Model file for the job. Use its own axes, mm. Face numbers are marked on the shaded views. A direction names the side the tool comes from. Give positions to 0.01 mm unless a question says otherwise; leave off trailing zeros. Loops run counter-clockwise (first coordinate to the right, second up) from the corner with the lowest first, then second, coordinate; pieces in that order, holes last. Notation, with made-up numbers: (-26.5, 46) - (17.5, 46) arc R16 cw to (17.5, 62) - close; hole circle Ø5 at (1, 59). An arc over 180 degrees is marked (long way). Answer as CSV lines item,"result". Start each with the question number.
Item 1: Pin check, flat tips, straight feed: pin 1 (3 mm diameter, centred on y = -2, z = -4.5, fed in from -X); pin 2 (4 mm diameter, centred on x = 16.5, y = -0.5, fed in from +Z); pin 3 (1 mm diameter, centred on y = -2, z = 3, fed in from +X). Stop position of each tip, or through.
Item 2: Drill centre lines: L1, parallel to X at y = -3.5, z = 3.75; L2, parallel to Y at x = 17.75, z = 1.25; L3, parallel to X at y = -12.5, z = -5.25. Where is each one in solid material? Low to high. Write a range as from..to.
Item 3: Tool access for the marked faces 4, 5, 6 and 7: list every direction of +Z, -Z, +X, -X, +Y, -Y with a clear straight run to the whole face (end or side of a thin tool).
Item 4: Pull direction Z, two halves, no side cores. Call the marked faces 1, 2 and 3: pulls with the +Z half, pulls with the -Z half, needs draft (parallel to the pull), parting line crosses it, or undercut.
Item 5: Saw through at A-A on y = -11.5. Give the cut face in (x, z), plus the area to 3 significant figures.
Item 6: Saw through at C-C on z = 3. Give the cut face in (x, y), plus the area to 3 significant figures.
Item 7: Saw through at B-B on x = 17.75. Give the cut face in (y, z).
Item 8: Saw through at D-D on y = 0. State how many separate pieces and enclosed holes the cut face has, plus the area to 3 significant figures.
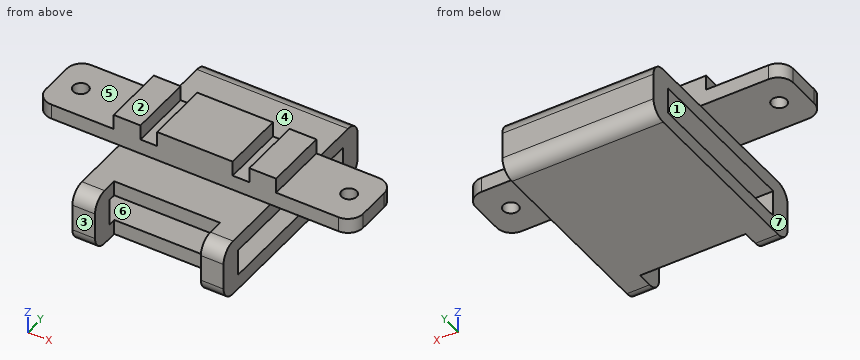
from build123d import *

# Parameters (mm, degrees)
SKETCH2_W           = 42
SKETCH2_H           = 8.4
BOSS_EXTRUDE1_DEPTH = 2
SKETCH3_W           = 3.55
SKETCH3_H           = 8.4
SKETCH3_W_2         = 10
BOSS_EXTRUDE2_DEPTH = 2
FILLET1_R           = 2
SKETCH4_R           = 1
CUT_EXTRUDE1_DEPTH  = 2
SKETCH5_W           = 20
SKETCH5_H           = 28
BOSS_EXTRUDE3_DEPTH = 7.5
FILLET2_R           = 2
SKETCH6_W           = 3.5
SKETCH6_H           = 22
CUT_EXTRUDE2_DEPTH  = 20
SKETCH7_W           = 14
SKETCH7_H           = 4
CUT_EXTRUDE3_DEPTH  = 10


with BuildPart() as part:
    # Sketch2 → Boss-Extrude1 (new body)
    with BuildSketch(Plane.XY):
        Rectangle(SKETCH2_W, SKETCH2_H)
    extrude(amount=BOSS_EXTRUDE1_DEPTH)

    # Sketch3 → Boss-Extrude2 (add)
    with BuildSketch(Plane.XY.offset(2)):
        with Locations((-8.975, 0)):
            Rectangle(SKETCH3_W, SKETCH3_H)
        with Locations((8.975, 0)):
            Rectangle(SKETCH3_W, SKETCH3_H)
        Rectangle(SKETCH3_W_2, SKETCH3_H)
    extrude(amount=BOSS_EXTRUDE2_DEPTH)

    # Fillet1
    fillet1_edges = [part.edges().sort_by_distance(p)[0] for p in [
        (-21, 4.2, 1),
        (21, 4.2, 1),
        (21, -4.2, 1),
        (-21, -4.2, 1),
    ]]
    fillet(fillet1_edges, radius=FILLET1_R)

    # Sketch4 → Cut-Extrude1 (cut)
    with BuildSketch(Plane.XY.offset(2)):
        with Locations((-17.75, 0)):
            Circle(SKETCH4_R)
        with Locations((17.75, 0)):
            Circle(SKETCH4_R)
    extrude(amount=-CUT_EXTRUDE1_DEPTH, mode=Mode.SUBTRACT)

    # Sketch5 → Boss-Extrude3 (add)
    with BuildSketch(Plane(origin=(0, 0, 0), x_dir=(-1, 0, 0), z_dir=(0, 0, -1))):
        Rectangle(SKETCH5_W, SKETCH5_H)
    extrude(amount=BOSS_EXTRUDE3_DEPTH)

    # Fillet2
    fillet2_edges = [part.edges().sort_by_distance(p)[0] for p in [
        (0, 14, 0),
        (0, -14, 0),
        (0, 14, -7.5),
        (0, -14, -7.5),
    ]]
    fillet(fillet2_edges, radius=FILLET2_R)

    # Sketch6 → Cut-Extrude2 (cut)
    with BuildSketch(Plane.ZY.offset(10)):
        with Locations((-3.75, 0)):
            Rectangle(SKETCH6_W, SKETCH6_H)
    extrude(amount=-CUT_EXTRUDE2_DEPTH, mode=Mode.SUBTRACT)

    # Sketch7 → Cut-Extrude3 (cut)
    with BuildSketch(Plane.XY):
        with Locations((0, -12)):
            Rectangle(SKETCH7_W, SKETCH7_H)
    extrude(amount=-CUT_EXTRUDE3_DEPTH, mode=Mode.SUBTRACT)


solid = part.part
Responses:
1,pin 1,"x = -10"
1,pin 2,"z = 2"
1,pin 3,"x = 10.75"
2,L1,"-10.75..-7.2, -5..5, 7.2..10.75"
2,L2,"-4.2..-1, 1..4.2"
2,L3,"-10..-7, 7..10"
3,face 4,"+Z, +X, -X, +Y"
3,face 5,"+Z, -X, +Y, -Y"
3,face 6,"+X, -X"
3,face 7,"-Z, -X, +Y, -Y"
4,face 1,"undercut"
4,face 2,"pulls with the +Z half"
4,face 3,"needs draft"
5,outline,"(-10, -7.5) - (-7, -7.5) - (-7, 0) - (-10, 0) - close; (7, -7.5) - (10, -7.5) - (10, 0) - (7, 0) - close"
5,area,"45.0 mm2"
6,outline,"(-10.75, -4.2) - (-7.2, -4.2) - (-7.2, 4.2) - (-10.75, 4.2) - close; (-5, -4.2) - (5, -4.2) - (5, 4.2) - (-5, 4.2) - close; (7.2, -4.2) - (10.75, -4.2) - (10.75, 4.2) - (7.2, 4.2) - close"
6,area,"144 mm2"
7,outline,"(-4.2, 0) - (-1, 0) - (-1, 2) - (-4.2, 2) - close; (1, 0) - (4.2, 0) - (4.2, 2) - (1, 2) - close"
8,separate pieces,"4"
8,enclosed holes,"0"
8,area,"190 mm2"
